```python
from build123d import *
from build123d import SkipClean  # not in build123d's __all__

# Parameters (mm, degrees)
F0_R     = 63.5
F2_DEPTH = 1270
F3_DEPTH = 1270
F4_DEPTH = 1270
F1_W     = 50.8
F1_H     = 127
F5_DEPTH = 1270
F6_DEPTH = 60.96


with BuildPart() as f2:
    # F0 (on Front) → F2 (new body, symmetric)
    with BuildSketch(Plane.XZ):
        Polygon((-228.6, 222.25), (-69.85, 222.25), (-47.625, 222.25), (-47.625, 241.3), (-250.825, 241.3), (-250.825, 222.25), align=None)
        with BuildLine():
            ThreePointArc((190.5, 0), (128.1457690484, 122.2758544982), (0, 171.45))
            Line((0, 171.45), (-44.45, 171.45))
            ThreePointArc((-44.45, 171.45), (-62.4105122421, 178.8894877579), (-69.85, 196.85))
            Line((-69.85, 196.85), (-69.85, 222.25))
            Line((-69.85, 222.25), (-228.6, 222.25))
            Line((-228.6, 222.25), (-228.6, 0))
            ThreePointArc((-228.6, 0), (-155.0557661778, -149.2358358304), (0, -209.55))
            ThreePointArc((0, -209.55), (135.7567353, -141.5993048182), (190.5, 0))
        make_face()
        with BuildLine():
            ThreePointArc((0, 171.45), (121.2334576344, 121.2334576344), (171.45, 0))
            ThreePointArc((171.45, 0), (-121.2334576344, -121.2334576344), (0, 171.45))
        make_face(mode=Mode.SUBTRACT)
        with BuildLine():
            ThreePointArc((0, 171.45), (-121.2334576344, -121.2334576344), (171.45, 0))
            ThreePointArc((171.45, 0), (121.2334576344, 121.2334576344), (0, 171.45))
        make_face()
        Circle(F0_R, mode=Mode.SUBTRACT)
        Circle(F0_R)
    extrude(amount=F2_DEPTH, both=True)

    # F1 (on Right) → F3 (intersect, symmetric)
    with BuildSketch(Plane.YZ):
        Polygon((-57.15, 222.25), (57.15, 222.25), (82.55, 222.25), (82.55, 241.3), (-82.55, 241.3), (-82.55, 222.25), align=None)
        Polygon((-57.15, -63.5), (-57.15, -209.55), (57.15, -209.55), (57.15, 222.25), (-57.15, 222.25), (-57.15, 63.5), align=None)
    extrude(amount=F3_DEPTH, both=True, mode=Mode.INTERSECT)



with BuildPart() as f4:
    # F0 (on Front) → F4 (new body, symmetric)
    with BuildSketch(Plane.XZ):
        Circle(F0_R)
    extrude(amount=F4_DEPTH, both=True)

    # F1 (on Right) → F5 (intersect, symmetric)
    with BuildSketch(Plane.YZ):
        with Locations((-82.55, 0)):
            Rectangle(F1_W, F1_H)
    extrude(amount=F5_DEPTH, both=True, mode=Mode.INTERSECT)


with BuildPart() as f2_1:
    add(f2.part, clean=False)

    with SkipClean():  # cleaning this boolean's faces spoils the solid; the shape is the same uncleaned
        add(f4.part)  # F6 merges F4
    # F0 (on Front) → F6 (join)
    with BuildSketch(Plane.XZ):
        with BuildLine():
            ThreePointArc((0, 171.45), (-121.2334576344, -121.2334576344), (171.45, 0))
            ThreePointArc((171.45, 0), (121.2334576344, 121.2334576344), (0, 171.45))
        make_face()
        Circle(F0_R, mode=Mode.SUBTRACT)
    with SkipClean():  # cleaning this boolean's faces spoils the solid; the shape is the same uncleaned
        extrude(amount=F6_DEPTH)


solid = f2_1.part
```
Verification items for the finished model (mm, model axes). A direction names the side the tool comes from. Give positions to 0.01 mm unless a question says otherwise; leave off trailing zeros. Write each loop counter-clockwise with the first axis right and the second up, starting at its lowest first coordinate (ties: lowest second). Pieces come first, ordered by that corner, then holes. Notation, with made-up numbers: M 53.5,1.25 L 75.5,1.25 A25 cw 75.5,34.25 Z; hole C 34,37 d7. An arc over 180 degrees is marked long. One line per question, with ' | ' between items.
1) Section check C-C on x = 97.5. Enter the section's corners in (y, z).
Result:
outline: M -60.96,-141.03 L -57.15,-141.03 L -57.15,-174.66 L 57.15,-174.66 L 57.15,144.78 L -57.15,144.78 L -57.15,141.03 L -60.96,141.03 Z
2) Gauge pin test, flat ends, axial feed: pin 1 Ø4 at (y, z) = (-81.5, -31.5) entering from -X; pin 2 Ø1 at (x, z) = (-120, 38) entering from +Y; pin 3 Ø1 at (x, y) = (116, 29.5) entering from +Z. Record the tip position at first contact, or that the pin passes through.
Result:
pin 1: stops at x = -56.23 | pin 2: stops at y = 57.15 | pin 3: stops at z = 132.71
3) Thickness scan on line 1 along Y through (x, z) = (-11, 52); line 2 along Z through (x, y) = (-2, -50); line 3 along Y through (x, z) = (-153, 186). Record the ranges inside material, lowest first. Write a range as [from, to].
Result:
line 1: y = [-107.95, 57.15] | line 2: z = [-209.54, 171.45] | line 3: y = [-57.15, 57.15]
4) Section check B-B on z = -10. Enter the section's corners in (x, y), plus the area to 3 significant figures.
Result:
outline: M -227.51,-57.15 L -171.16,-57.15 L -171.16,-60.96 L -62.71,-60.96 L -62.71,-107.95 L 62.71,-107.95 L 62.71,-60.96 L 171.16,-60.96 L 171.16,-57.15 L 190.26,-57.15 L 190.26,57.15 L -227.51,57.15 Z | area: 54,900 mm2
5) Mould release check, pull along Z, two halves, no side actions. Record for faces 6 (the flat face through (-151, 72, 222.25)), 7 (the cylindrical face through (129.6, -0.8, 120.954)), 8 (the flat face through (-250.825, -1, 232)): released by +Z, released by -Z, zero draft, split by the parting line, or undercut.
Result:
face 6: undercut | face 7: released by +Z | face 8: zero draft
6) Section check D-D on z = 162. Enter the section's corners in (x, y), plus the area to 3 significant figures.
Result:
outline: M -228.6,-57.15 L -56.13,-57.15 L -56.13,-60.96 L 56.13,-60.96 L 56.13,-57.15 L 59.42,-57.15 L 59.42,57.15 L -228.6,57.15 Z | area: 33,300 mm2
7) Set-up check for faces 1 (the flat face through (-69.85, -1, 209)), 2 (the flat face through (74, -60.96, 2)), 3 (the flat face through (-22, -1, 171.45)), 4 (the flat face through (-16, 57.15, 3)), 5 (the flat face through (-228.6, -1, 113)): record each of +Z, -Z, +X, -X, +Y, -Y from which the full face is reachable in a straight line by a thin tool's end or side.
Result:
face 1: +X, +Y, -Y | face 2: -Y | face 3: +Z, +X, +Y, -Y | face 4: -Z, +X, -X, +Y | face 5: -Z, -X, +Y, -Y
